Check sheet for the modelled part. Datum: model origin and axes. Units: mm. Face numbers are marked on the shaded views. A direction names the side the tool comes from. Round coordinates to 2 decimals unless told otherwise and drop trailing zeros. Loops run counter-clockwise (first coordinate to the right, second up) from the corner with the lowest first, then second, coordinate; pieces in that order, holes last. Notation, with made-up numbers: (49.5, 62) - (60.5, 62) arc R21 cw to (60.5, 73) - close; hole circle Ø7 at (62, 40.25). An arc over 180 degrees is marked (long way). Put each result on its own line as item: value.
```python
from build123d import *

# Parameters (mm, degrees)
BASE_FLANGE1_DEPTH         = 4.7625
CUT_EXTRUDE1_DEPTH         = 532.464280138
F_5_2_5_2_DIAMETER_HOLE1_D = 5.2
F_4_2_4_2_DIAMETER_HOLE1_D = 4.2


# Sheet-metal steps are written as plain solids
with BuildPart() as part:
    # Sketch11 → Base-Flange1 (new body)
    with BuildSketch(Plane.XZ.offset(-2274.861409739)):
        with BuildLine():
            Line((-14.848279171, -526.663757324), (-14.848279171, -524.922409256))
            ThreePointArc((-14.848279171, -524.922409256), (-14.061019769, -522.229303864), (-11.947152511, -520.384267488))
            ThreePointArc((-11.947152511, -520.384267488), (-9.635257269, -518.200933677), (-9.1073955, -515.065145404))
            Line((-9.1073955, -515.065145404), (-13.536920305, -487.054470663))
            ThreePointArc((-13.536920305, -487.054470663), (-18.839332617, -478.263515672), (-24.167937573, -487.038618817))
            Line((-24.167937573, -487.038618817), (-28.703176429, -515.010971128))
            ThreePointArc((-28.703176429, -515.010971128), (-28.167792512, -518.185746554), (-25.8079527, -520.375949969))
            ThreePointArc((-25.8079527, -520.375949969), (-23.652946505, -522.220569615), (-22.848279171, -524.940713697))
            Line((-22.848279171, -524.940713697), (-22.848279171, -526.663757324))
            ThreePointArc((-22.848279171, -526.663757324), (-18.848279171, -530.663757324), (-14.848279171, -526.663757324))
        make_face()
    extrude(amount=-BASE_FLANGE1_DEPTH)

    # Sketch16 → Cut-Extrude1 (cut, through all)
    with BuildSketch(Plane(origin=(0, 2279.623909739, 0), x_dir=(-1, 0, 0), z_dir=(0, 1, 0))):
        with BuildLine():
            ThreePointArc((23.232934356, -511.51957962), (18.659918541, -512.162345688), (14.104175105, -511.406816996))
            ThreePointArc((14.104175105, -511.406816996), (10.671023737, -513.070256662), (12.334463403, -516.50340803))
            ThreePointArc((12.334463403, -516.50340803), (18.94176187, -517.91323157), (25.531859334, -516.425074701))
            ThreePointArc((25.531859334, -516.425074701), (26.835144386, -512.822864672), (23.232934356, -511.51957962))
        make_face()
    extrude(amount=-CUT_EXTRUDE1_DEPTH, mode=Mode.SUBTRACT)

    # Ø5.2 (5.2) Diameter Hole1 (through all)
    with Locations(Plane(origin=(0, 2279.623909739, 0), x_dir=(1, 0, 0), z_dir=(0, 1, 0))):
        with Locations((-18.848279171, 484.263509002)):
            Hole(F_5_2_5_2_DIAMETER_HOLE1_D / 2)

    # Ø4.2 (4.2) Diameter Hole1 (through all)
    with Locations(Plane(origin=(0, 2279.623909739, 0), x_dir=(1, 0, 0), z_dir=(0, 1, 0))):
        with Locations((-18.848279171, 499.538509002), (-18.848279171, 527.163757324)):
            Hole(F_4_2_4_2_DIAMETER_HOLE1_D / 2)


solid = part.part
```
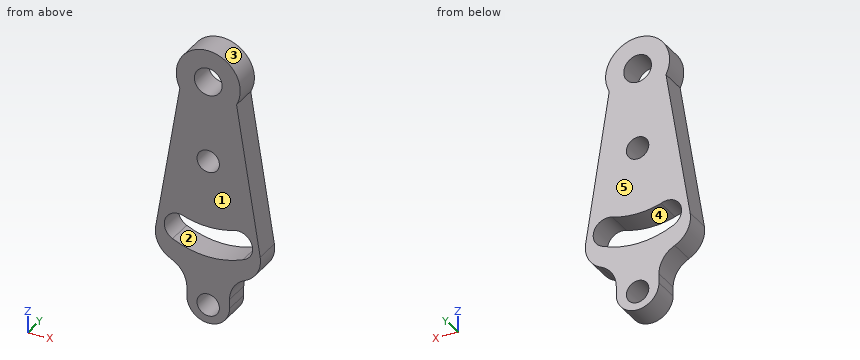
Item 1: Section check D-D on x = -15.5. Enter the section's corners in (y, z).
Filled sheet:
outline: (2274.86, -528.85) - (2279.62, -528.85) - (2279.62, -517.55) - (2274.86, -517.55) - close; (2274.86, -511.79) - (2279.62, -511.79) - (2279.62, -479.28) - (2274.86, -479.28) - close
Item 2: Go/stop test with flat-tipped pins: pin 1 (1.4 mm diameter, centred on y = 2278, z = -526, fed in from -X); pin 2 (0.9 mm diameter, centred on y = 2276.5, z = -526, fed in from +X). Record where each tip stops, or that it passes through.
Filled sheet:
pin 1: x = -22.85
pin 2: x = -14.85
Item 3: Section check B-B on x = -18. Enter the section's corners in (y, z), then the cut area to 3 significant figures.
Filled sheet:
outline: (2274.86, -530.57) - (2279.62, -530.57) - (2279.62, -529.08) - (2274.86, -529.08) - close; (2274.86, -525.24) - (2279.62, -525.24) - (2279.62, -517.89) - (2274.86, -517.89) - close; (2274.86, -512.14) - (2279.62, -512.14) - (2279.62, -501.46) - (2274.86, -501.46) - close; (2274.86, -497.62) - (2279.62, -497.62) - (2279.62, -486.72) - (2274.86, -486.72) - close; (2274.86, -481.81) - (2279.62, -481.81) - (2279.62, -478.32) - (2274.86, -478.32) - close
area: 161 mm²
Item 4: Tool access check on the marked faces 1 and 2. Record the directions out of +Z, -Z, +X, -X, +Y, -Y that give a thin tool (end or side, any length) a straight path to the whole face; none if there is none.
Filled sheet:
face 1: +Z, -Z, +X, -X, -Y
face 2: +Y, -Y
Item 5: Thickness scan on line 1 (Z direction, x = -17.5, y = 2276.1); line 2 (Z direction, x = -20.75, y = 2278.85); line 3 (Z direction, x = -16.5, y = 2279). Record the ranges inside material, lowest first. Write a range as from..to.
Filled sheet:
line 1: -530.43..-528.77, -525.55..-517.86, -512.1..-501.15, -497.93..-486.49, -482.04..-478.42
line 2: -530.18..-528.05, -526.27..-517.8, -512.04..-500.43, -498.65..-486.04, -482.49..-478.57
line 3: -529.9..-517.74, -511.98..-485.38, -483.15..-478.74
Item 6: Section check A-A on z = -517. Enter the section's corners in (x, y), then the cut area to 4 significant figures.
Filled sheet:
outline: (-28.62, 2274.86) - (-24.13, 2274.86) - (-24.13, 2279.62) - (-28.62, 2279.62) - close; (-13.56, 2274.86) - (-9.18, 2274.86) - (-9.18, 2279.62) - (-13.56, 2279.62) - close
area: 42.25 mm²
Item 7: Release check for a two-part mould opening along X. For the marked faces 3, 4 and 5 record: +X half, -X half, draft (parallel to the pull), parting line (faces both ways), or undercut.
Filled sheet:
face 3: parting line
face 4: undercut
face 5: draft
Item 8: Section check C-C on y = 2278. Enter the section's corners in (x, z).
Filled sheet:
outline: (-28.7, -515.01) arc R5 ccw to (-25.81, -520.38) arc R5 cw to (-22.85, -524.94) - (-22.85, -526.66) arc R4 ccw to (-14.85, -526.66) - (-14.85, -524.92) arc R5 cw to (-11.95, -520.38) arc R5 ccw to (-9.11, -515.07) - (-13.54, -487.05) arc R6 ccw (long way) to (-24.17, -487.04) - close; hole (-25.53, -516.43) arc R15.75 ccw to (-12.33, -516.5) arc R2.7 ccw to (-14.1, -511.41) arc R15.25 cw to (-23.23, -511.52) arc R2.71 ccw to start; hole circle Ø5.2 at (-18.85, -484.26); hole circle Ø4.2 at (-18.85, -527.16); hole circle Ø4.2 at (-18.85, -499.54)
